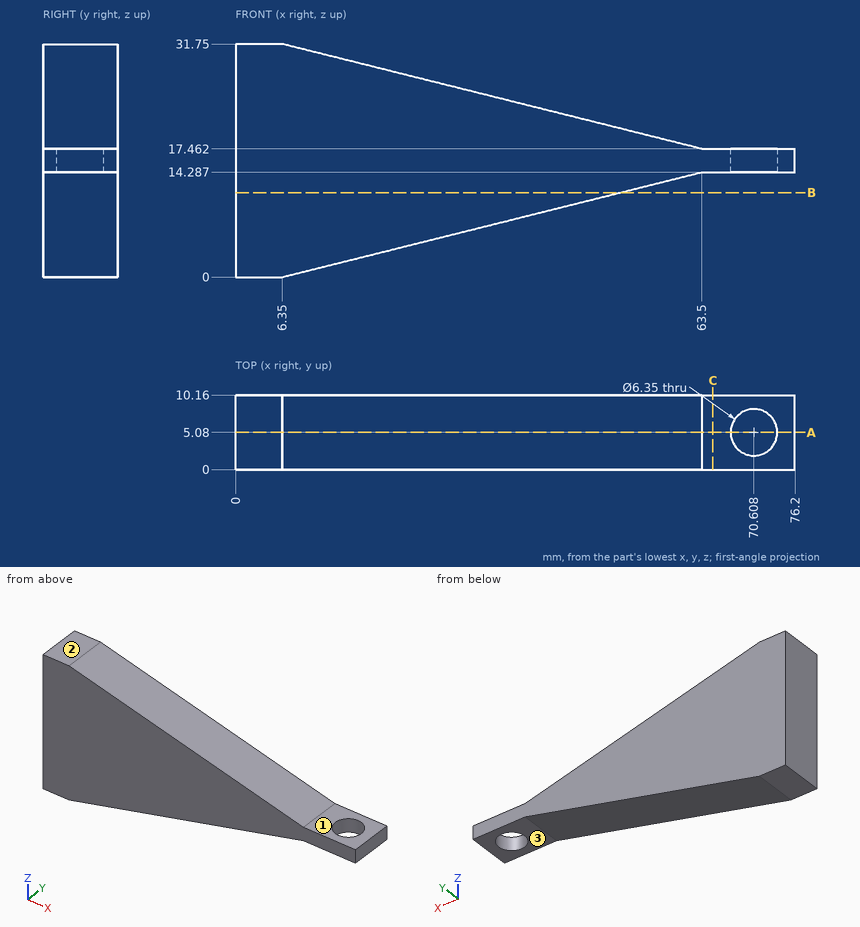
Print and shaded views of the part. All mm, measured from the part's lowest x, y and z. A direction names the side the tool comes from. Coordinates: 2 decimals unless noted, no trailing zeros. Order: outer loops, then holes, each group sorted by start corner. A loop starts at its lowest first (then second) coordinate and runs counter-clockwise, first axis right, second up. Notation, with made-up numbers: M 26.5,56.25 L 70.5,56.25 A23 ccw 70.5,75.25 Z; hole C 54.5,84 d2. An arc over 180 degrees is marked long. One line per question, with ' | ' between items. Start each with the question number.
Q1. Flat gauge pins, fed straight in: pin 1 Ø5 at (x, y) = (72, 5) entering from +Z; pin 2 Ø2 at (x, y) = (47.5, 7.5) entering from +Z. Where does each tip first touch, or does it go through?
Q2. Saw through at B-B (z = 11.5). List the corners of the cut face in (x, y).
Q3. 3-axis set-ups, long thin cutter, end or side, ignore diameter. For the marked faces 1, 2 and 3: which of +Z, -Z, +X, -X, +Y, -Y reach the whole face in a straight line?
Q4. Probe L1, parallel to X at y = 5, z = 15; L2, parallel to Z at x = 37, y = 9.75; L3, parallel to Z at x = 72, y = 1.5. List the from-to ranges inside material, lowest first. Write a range as from..to.
Q5. Saw through at C-C (x = 65). List the corners of the cut face in (y, z).
Q6. Saw through at A-A (y = 5.08). List the corners of the cut face in (x, z), then the cut area to 3 significant figures.
Check values:
1) pin 1: stops at z = 17.46 | pin 2: stops at z = 21.71
2) outline: M 0,0 L 52.35,0 L 52.35,10.16 L 0,10.16 Z
3) face 1: +Z, +X, +Y, -Y | face 2: +Z, +X, -X, +Y, -Y | face 3: -Z, +X, +Y, -Y
4) L1: x = 0..67.43, 73.78..76.2 | L2: z = 7.66..24.09 | L3: z = 14.29..17.46
5) outline: M 0,14.29 L 10.16,14.29 L 10.16,17.46 L 0,17.46 Z
6) outline: M 0,0 L 6.35,0 L 63.5,14.29 L 67.43,14.29 L 67.43,17.46 L 63.5,17.46 L 6.35,31.75 L 0,31.75 Z; M 73.78,14.29 L 76.2,14.29 L 76.2,17.46 L 73.78,17.46 Z | area: 1,220 mm2
